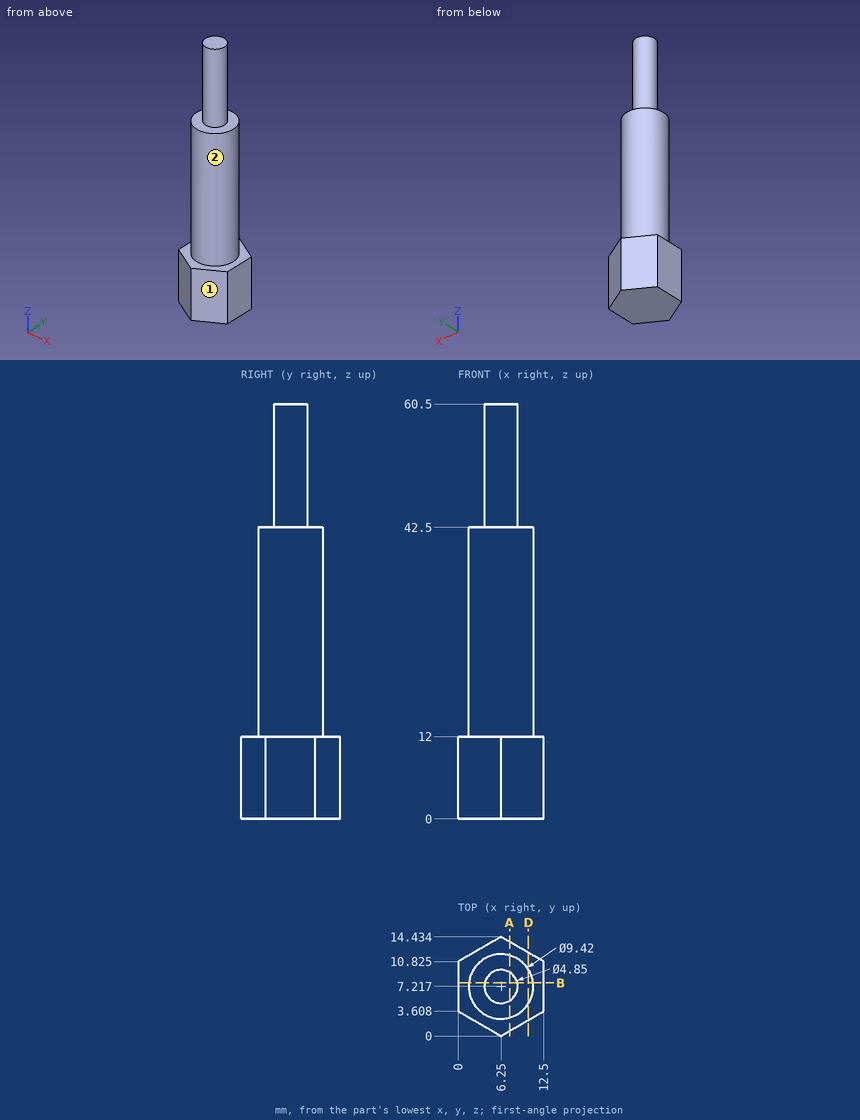
Study the drawing (mm; zero at the part's minimum x, y, z) and answer. A direction names the side the tool comes from. Give positions to 0.01 mm unless a question says otherwise; leave off trailing zeros. Loops run counter-clockwise (first coordinate to the right, second up) from the corner with the lowest first, then second, coordinate; pieces in that order, holes last. Notation, with made-up numbers: (63, -25.5) -> (86, -25.5) arc R20 ccw to (86, 4.5) -> close; hole circle Ø9 at (25.5, 5.25). An arc over 180 degrees is marked (long way). Use a Markdown table: item, result. Add a question column.
1) The part is cut by section B-B, the plane y = 7.75. Determine the outline of the cut face in (x, z) (1 decimal).
2) The part is cut by section A-A, the plane x = 7.5. Determine the outline of the cut face in (y, z) (1 decimal), plus the area to 3 significant figures.
3) Which of the six approach directions +Z, -Z, +X, -X, +Y, -Y give full straight-line access (tool end or side, diameter ignored) to the marked faces 1 and 2?
4) The part is cut by section D-D, the plane x = 10.25. Determine the outline of the cut face in (y, z) (1 decimal).
5) Each of these flat-tipped pins is pushed along its axis until it touches: P1, Ø6, axis at x = 4, z = 52, coming from the +Y side; P2, Ø1.5, axis at x = 4.5, z = 47.5, coming from the -Y side. Where does it stop, or does it pass through?
6) Consider line 1 along Z through (x, y) = (11.25, 7.5); line 2 along Z through (x, y) = (3.25, 4.5); line 3 along Y through (x, z) = (6.5, 44) (1 decimal). Determine where each line is inside the solid, lowest interval first.
Reported:
| question | item | result |
|---|---|---|
| 1 | outline | (0, 0) -> (12.5, 0) -> (12.5, 12) -> (10.9, 12) -> (10.9, 42.5) -> (8.6, 42.5) -> (8.6, 60.5) -> (3.9, 60.5) -> (3.9, 42.5) -> (1.6, 42.5) -> (1.6, 12) -> (0, 12) -> close |
| 2 | outline | (0.7, 0) -> (13.7, 0) -> (13.7, 12) -> (11.8, 12) -> (11.8, 42.5) -> (9.3, 42.5) -> (9.3, 60.5) -> (5.1, 60.5) -> (5.1, 42.5) -> (2.7, 42.5) -> (2.7, 12) -> (0.7, 12) -> close |
| 2 | area | 508 mm^2 |
| 3 | face 1 | +Z, -Z, +X, -Y |
| 3 | face 2 | +Z |
| 4 | outline | (2.3, 0) -> (12.1, 0) -> (12.1, 12) -> (9.7, 12) -> (9.7, 42.5) -> (4.7, 42.5) -> (4.7, 12) -> (2.3, 12) -> close |
| 5 | P1 | stops at y = 9.64 |
| 5 | P2 | stops at y = 5.01 |
| 6 | line 1 | z = 0 to 12 |
| 6 | line 2 | z = 0 to 42.5 |
| 6 | line 3 | y = 4.8 to 9.6 |
